The listing builds one solid part. Answer for the finished solid, in the listing's coordinates (mm). Face numbers are marked on the shaded views. A direction names the side the tool comes from. Round coordinates to 2 decimals unless told otherwise and drop trailing zeros. Order: outer loops, then holes, each group sorted by start corner. A loop starts at its lowest first (then second) coordinate and runs counter-clockwise, first axis right, second up. Notation, with made-up numbers: M 25.5,-16.5 L 42.5,-16.5 A17 ccw 42.5,6.5 Z; hole C 59,82 d11. An arc over 180 degrees is marked long. Write item = value, one per line. Start each with the question number.
(1) A cutting plane is placed at C-C, the plane z = -0.5. Determine the outline of the cut face in (x, y), and give its area (3 significant figures).
(2) Which of the six approach directions +Z, -Z, +X, -X, +Y, -Y give full straight-line access (tool end or side, diameter ignored) to the marked faces 1 and 2?
(3) Straight lines are drawn through the part: probe 1 along Z at (x, y) = (27.5, 2); probe 2 along X at (y, z) = (4.75, -12.5); probe 3 along Y at (x, z) = (8, 4.5). For each, find the intervals that lie inside material, in ascending order. Write a range as from..to.
(4) A cutting plane is placed at D-D, the plane z = -13. Determine the outline of the cut face in (x, y).
(5) For a pull along Z with two mould halves and no side action, classify the marked faces 3, 4 and 5 as released by +Z, released by -Z, zero draft, split by the parting line, or undercut.
(6) A cutting plane is placed at B-B, the plane x = 30. Determine the outline of the cut face in (y, z), and give its area (3 significant figures).
(7) Each of these flat-tipped pins is pushed along its axis until it touches: pin 1 (1.5 mm diameter, centred on x = 72, y = 1.5, fed in from -Z); pin 2 (4 mm diameter, centred on x = 84, y = 2.5, fed in from +Z); pin 3 (12 mm diameter, centred on x = 62, z = -12, fed in from +Y); pin 4 (10 mm diameter, centred on x = 110, z = -3.5, fed in from -Y). Where does it stop, or does it pass through?
(8) A cutting plane is placed at A-A, the plane y = 3.5. Determine the outline of the cut face in (x, z), and give its area (3 significant figures).
from build123d import *

# Parameters (mm, degrees)
EXTRUDE_1_DEPTH     = 13
EXTRUDE_2_DEPTH     = 5
CUT_EXTRUDE_1_DEPTH = 140.061137634


with BuildPart() as part:
    # Sketch 1 → Extrude 1 (new body)
    with BuildSketch(Plane(origin=(0, 0, 0), x_dir=(1, 0, 0), z_dir=(0, 1, 0))):
        with BuildLine():
            Line((137, 0), (122, 0))
            Line((122, 0), (122, -3.83772234))
            ThreePointArc((122, -3.83772234), (122.177358944, -4.853939575), (122.68846498, -5.75))
            ThreePointArc((122.68846498, -5.75), (123.722665467, -6.55220507), (125, -6.83772234))
            Line((125, -6.83772234), (125.5, -6.83772234))
            ThreePointArc((125.5, -6.83772234), (126.882997438, -7.175520603), (127.954545455, -8.112843616))
            ThreePointArc((127.954545455, -8.112843616), (129.429754152, -11.909474928), (128.969252111, -15.956521739))
            ThreePointArc((128.969252111, -15.956521739), (129.319163119, -18.713120722), (131.781929326, -20))
            Line((131.781929326, -20), (134, -20))
            ThreePointArc((134, -20), (136.121320344, -19.121320344), (137, -17))
            Line((137, -17), (137, 0))
        make_face()
        with BuildLine():
            Line((122, 3.83772234), (122, 0))
            Line((122, 0), (137, 0))
            Line((137, 0), (137, 17))
            ThreePointArc((137, 17), (136.121320344, 19.121320344), (134, 20))
            Line((134, 20), (131.781929326, 20))
            ThreePointArc((131.781929326, 20), (129.319163119, 18.713120722), (128.969252111, 15.956521739))
            ThreePointArc((128.969252111, 15.956521739), (129.429754152, 11.909474928), (127.954545455, 8.112843616))
            ThreePointArc((127.954545455, 8.112843616), (126.882997438, 7.175520603), (125.5, 6.83772234))
            Line((125.5, 6.83772234), (125, 6.83772234))
            ThreePointArc((125, 6.83772234), (123.722665467, 6.55220507), (122.68846498, 5.75))
            ThreePointArc((122.68846498, 5.75), (122.177358944, 4.853939575), (122, 3.83772234))
        make_face()
    extrude(amount=EXTRUDE_1_DEPTH)

    # Sketch 1_3 → Extrude 2 (add)
    with BuildSketch(Plane(origin=(0, 0, 0), x_dir=(1, 0, 0), z_dir=(0, 1, 0))):
        with BuildLine():
            Line((0, 5.75), (0, 0))
            Line((0, 0), (122, 0))
            Line((122, 0), (122, 3.83772234))
            ThreePointArc((122, 3.83772234), (122.177358944, 4.853939575), (122.68846498, 5.75))
            Line((122.68846498, 5.75), (0, 5.75))
        make_face()
        with BuildLine():
            Line((122, 0), (0, 0))
            Line((0, 0), (0, -5.75))
            Line((0, -5.75), (122.68846498, -5.75))
            ThreePointArc((122.68846498, -5.75), (122.177358944, -4.853939575), (122, -3.83772234))
            Line((122, -3.83772234), (122, 0))
        make_face()
    extrude(amount=EXTRUDE_2_DEPTH)

    # Sketch 2 → Cut-Extrude 1 (cut, through all)
    with BuildSketch(Plane(origin=(137, 0, 0), x_dir=(0, 0, -1), z_dir=(1, 0, 0))):
        with BuildLine():
            Line((-11.193056067, 13), (11.193056067, 13))
            ThreePointArc((11.193056067, 13), (7.438767237, 12.422890395), (4.031140189, 10.74485046))
            ThreePointArc((4.031140189, 10.74485046), (3.317442984, 10.041838714), (2.875, 9.143043175))
            ThreePointArc((2.875, 9.143043175), (0, 7), (-2.875, 9.143043175))
            ThreePointArc((-2.875, 9.143043175), (-3.317442984, 10.041838714), (-4.031140189, 10.74485046))
            ThreePointArc((-4.031140189, 10.74485046), (-7.438767237, 12.422890395), (-11.193056067, 13))
        make_face()
    extrude(amount=-CUT_EXTRUDE_1_DEPTH, mode=Mode.SUBTRACT)


solid = part.part
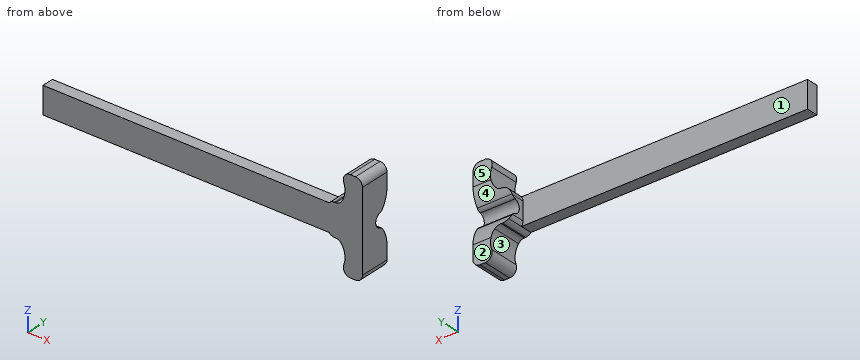
Reported:
q1.outline = M 0,0 L 137,0 L 137,7.04 L 122,7.04 L 122,5 L 0,5 Z
q1.area = 716 mm²
q2.face_1 = +Z, -Z, -X, +Y
q2.face_2 = +Z, -Z, +X, -X, +Y
q3.probe_1 = -5.75..5.75
q3.probe_2 = 129.49..137
q3.probe_3 = 0..5
q4.outline = M 129.5,0 L 137,0 L 137,13 L 129.5,13 Z
q5.face_3 = undercut
q5.face_4 = undercut
q5.face_5 = zero draft
q6.outline = M 0,-5.75 L 5,-5.75 L 5,5.75 L 0,5.75 Z
q6.area = 57.5 mm²
q7.pin_1 = -5.75
q7.pin_2 = 5.75
q7.pin_3 = through
q7.pin_4 = 0
q8.outline = M 0,-5.75 L 122.69,-5.75 A3 ccw 125,-6.84 L 125.5,-6.84 A3 cw 127.95,-8.11 A8.5 cw 128.97,-15.96 A3 ccw 131.78,-20 L 134,-20 A3 ccw 137,-17 L 137,17 A3 ccw 134,20 L 131.78,20 A3 ccw 128.97,15.96 A8.5 cw 127.95,8.11 A3 cw 125.5,6.84 L 125,6.84 A3 ccw 122.69,5.75 L 0,5.75 Z
q8.area = 1,810 mm²
